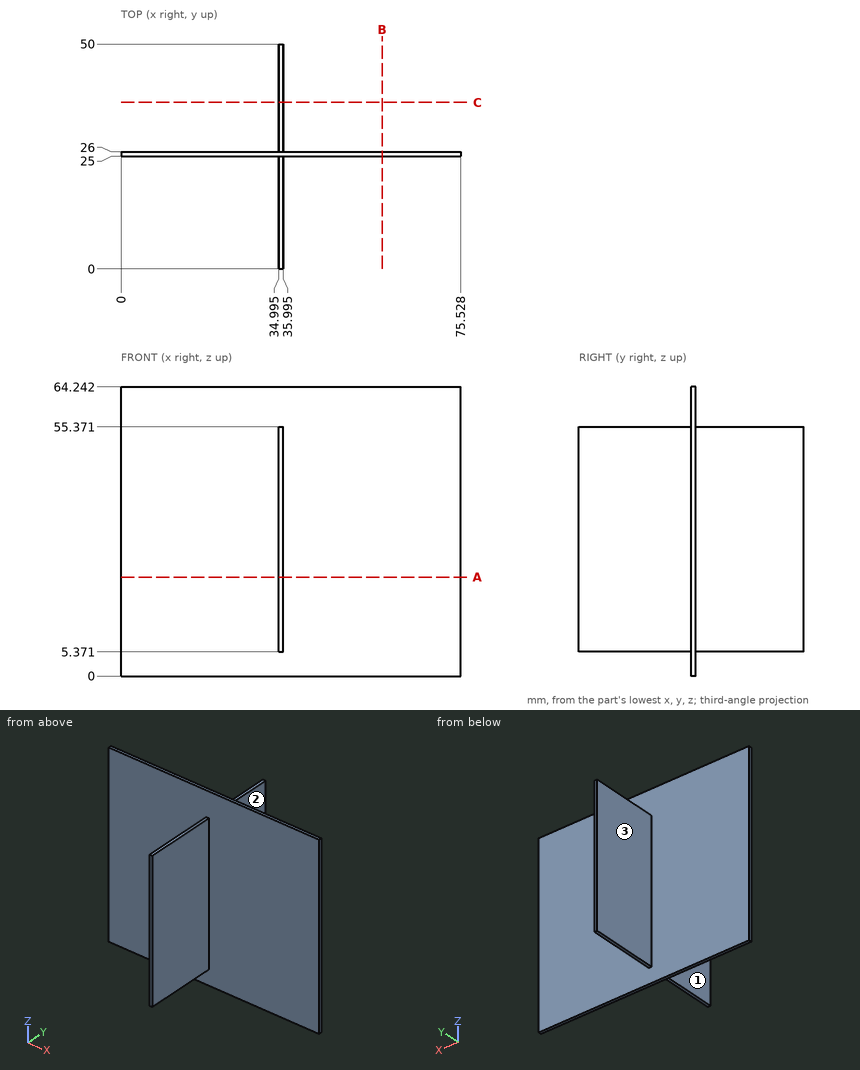
Job drawing, mm, ordinate dimensions from the low corner. One solid piece. A direction names the side the tool comes from. Give positions to 0.01 mm unless a question says otherwise; leave off trailing zeros. Order: outer loops, then holes, each group sorted by start corner. A loop starts at its lowest first (then second) coordinate and runs counter-clockwise, first axis right, second up. Notation, with made-up numbers: (19, -30.75) - (31, -30.75) arc R25 cw to (31, 5.25) - close; hole circle Ø1 at (-38, 78.5). An arc over 180 degrees is marked (long way). Return JSON: item names as keys, results as strings.
1) Cut at B-B, the plane x = 58. Give the cut face in (y, z).
Geometry says:
{"outline": "(25, 0) - (26, 0) - (26, 64.24) - (25, 64.24) - close"}
2) Probe line 1 (Y direction, x = 21.5, z = 56); line 2 (X direction, y = 22.5, z = 34.5) (1 decimal); line 3 (Z direction, x = 35.5, y = 42). List the from-to ranges inside material, lowest first. Write a range as from..to.
Geometry says:
{"line 1": "25..26", "line 2": "35..36", "line 3": "5.37..55.37"}
3) Cut at A-A, the plane z = 22. Give the cut face in (x, y) (1 decimal).
Geometry says:
{"outline": "(0, 25) - (35, 25) - (35, 0) - (36, 0) - (36, 25) - (75.5, 25) - (75.5, 26) - (36, 26) - (36, 50) - (35, 50) - (35, 26) - (0, 26) - close"}
4) Cut at C-C, the plane y = 37. Give the cut face in (x, z) (1 decimal).
Geometry says:
{"outline": "(35, 5.4) - (36, 5.4) - (36, 55.4) - (35, 55.4) - close"}
5) Flat gauge pins, fed straight in: P1, Ø1.5, axis at x = 55, z = 24.5, coming from the -Y side; P2, Ø0.8, axis at x = 35.5, y = 15, coming from the +Z side; P3, Ø20, axis at y = 11.5, z = 25.5, coming from the +X side (1 decimal); P4, Ø4, axis at x = 54, y = 29.5, coming from the -Z side. Where does each tip first touch, or does it go through?
Geometry says:
{"P1": "y = 25", "P2": "z = 55.37", "P3": "x = 36", "P4": "through"}
6) 3-axis set-ups, long thin cutter, end or side, ignore diameter. For the marked faces 1, 2 and 3: which of +Z, -Z, +X, -X, +Y, -Y reach the whole face in a straight line?
Geometry says:
{"face 1": "+Z, -Z, -X, -Y", "face 2": "+Z, -Z, +X, +Y", "face 3": "+Z, -Z, -X, +Y"}
